```python
from build123d import *

# Parameters (mm, degrees)
EXTRUDE_1_DEPTH = 5


with BuildPart() as part:
    # 草图1 → 凸台-拉伸1 (new body)
    with BuildSketch(Plane.XY):
        with BuildLine():
            Line((8.992179856, 1.5), (10, 1.5))
            Line((10, 1.5), (10, 0))
            Line((10, 0), (0, 0))
            Line((0, 0), (0, 1.5))
            Line((0, 1.5), (1.007820144, 1.5))
            ThreePointArc((1.007820144, 1.5), (-1.893270413, 6.032287794), (-0.720584593, 11.284217633))
            Line((-0.720584593, 11.284217633), (1.492224546, 11.806096066))
            ThreePointArc((1.492224546, 11.806096066), (4.953081958, 1.500191421), (8.581658268, 11.748246776))
            Line((8.581658268, 11.748246776), (10.744690333, 11.249816618))
            ThreePointArc((10.744690333, 11.249816618), (11.889585712, 6.011610437), (8.992179856, 1.5))
        make_face()
    extrude(amount=EXTRUDE_1_DEPTH)


solid = part.part
```
Source: CAD feature listing. Evaluate the final solid. Frame: model axes, mm. A direction names the side the tool comes from. Round coordinates to 2 decimals unless told otherwise and drop trailing zeros. Write each loop counter-clockwise with the first axis right and the second up, starting at its lowest first coordinate (ties: lowest second). Pieces come first, ordered by that corner, then holes. Notation, with made-up numbers: M 68,30.25 L 98,30.25 A20 cw 98,52.25 Z; hole C -21,-21.5 d5. An arc over 180 degrees is marked long. Answer as a JSON object with one key per item and string values. Group by question number.
(1) Section query A-A on y = 9. Output: boundary loops of the cut face in (x, z).
(2) Ray query, line 1 (X direction, y = 7.25, z = 3.05); line 2 (Y direction, x = 5, z = 3.3); line 3 (X direction, y = 0.5, z = 0.3). Return the intervals inside material, ascending. Write a range as [from, to].
(3) Section query D-D on x = 5. Output: boundary loops of the cut face in (y, z), then the cut area to 3 significant figures.
(4) Mould query, pull axis Y, two halves, no side actions, for faces 3 (the flat face through (10, 1, 2)), 4 (the flat face through (5, 0, 2)), 5 (the cylindrical face through (4.754, 1.505, 2.465)). Classes: +Y half, -Y half, draft (parallel to the pull), parting line (faces both ways), or undercut.
(5) First-contact query: pin 1 (4 mm diameter, centred on x = 1.5, y = 3.5, fed in from -Z); pin 2 (1.6 mm diameter, centred on y = 1, z = 2, fed in from -X); pin 3 (0.8 mm diameter, centred on x = 9.5, z = 2, fed in from +Y); pin 4 (1.1 mm diameter, centred on x = 0.5, z = 3.5, fed in from +Y). Flat tips, straight axial feed; report the tip coordinate or a pass-through.
(6) Reachability of faces 1 (the flat face through (5, 1, 0)), 2 (the flat face through (0, 1, 2)) from +Z, -Z, +X, -X, +Y, -Y: full face, straight path, thin tool, end or side. Return the list, or none.
(7) Section query C-C on y = 7.25. Output: boundary loops of the cut face in (x, z).
(8) Section query B-B on z = 3. Output: boundary loops of the cut face in (x, y), then the cut area to 3 significant figures.
Computed values:
{
 "1": {"outline": "M -1.78,0 L -0.48,0 L -0.48,5 L -1.78,5 Z; M 10.48,0 L 11.78,0 L 11.78,5 L 10.48,5 Z"},
 "2": {"line 1": "[-2, -0.75], [10.75, 12]", "line 2": "[0, 1.5]", "line 3": "[0, 10]"},
 "3": {"outline": "M 0,0 L 1.5,0 L 1.5,5 L 0,5 Z", "area": "7.50 mm^2"},
 "4": {"face 3": "draft", "face 4": "-Y half", "face 5": "undercut"},
 "5": {"pin 1": "z = 0", "pin 2": "x = 0", "pin 3": "y = 11.63", "pin 4": "y = 11.7"},
 "6": {"face 1": "-Z, +X, -X, +Y, -Y", "face 2": "+Z, -Z, -X, -Y"},
 "7": {"outline": "M -2,0 L -0.75,0 L -0.75,5 L -2,5 Z; M 10.75,0 L 12,0 L 12,5 L 10.75,5 Z"},
 "8": {"outline": "M -0.72,11.28 A7 ccw 1.01,1.5 L 0,1.5 L 0,0 L 10,0 L 10,1.5 L 8.99,1.5 A7 ccw 10.74,11.25 L 8.58,11.75 A5.75 cw long 1.49,11.81 Z", "area": "44.9 mm^2"}
}
